CAD build for the part. Positions are in the model's coordinates, mm. Face numbers are marked on the shaded views. A direction names the side the tool comes from. Round coordinates to 2 decimals unless told otherwise and drop trailing zeros. Order: outer loops, then holes, each group sorted by start corner. A loop starts at its lowest first (then second) coordinate and runs counter-clockwise, first axis right, second up. Notation, with made-up numbers: M -23.5,84 L 12.5,84 A20 ccw 12.5,99 Z; hole C 4,4.5 d3. An arc over 180 degrees is marked long. Answer as a JSON object with one key per item and string values. Group by question number.
```python
from build123d import *

# Parameters (mm, degrees)
EXTRUDE_1_DEPTH     = 12.1
SKETCH_3_R          = 6.05
EXTRUDE_2_DEPTH     = 4.3
SKETCH_4_R          = 2.43
EXTRUDE_3_DEPTH     = 4
SKETCH_5_R          = 1.1
CUT_EXTRUDE_1_DEPTH = 4


with BuildPart() as part:
    # Эскиз1 → Бобышка-Вытянуть1 (new body)
    with BuildSketch(Plane.XY):
        Polygon((0, 0), (22.5, 0), (22.5, 15.7), (27.4, 15.7), (27.4, 18.2), (22.5, 18.2), (22.5, 22.4), (0, 22.4), (0, 18.2), (-4.9, 18.2), (-4.9, 15.7), (0, 15.7), align=None)
    extrude(amount=EXTRUDE_1_DEPTH)

    # Эскиз3 → Бобышка-Вытянуть2 (add)
    with BuildSketch(Plane(origin=(0, 22.4, 0), x_dir=(1, 0, 0), z_dir=(0, 1, 0))):
        with Locations(Location((16.45, -6.05, 0), (0, 0, 270))):
            Circle(SKETCH_3_R)
    extrude(amount=EXTRUDE_2_DEPTH)

    # Эскиз4 → Бобышка-Вытянуть3 (add)
    with BuildSketch(Plane(origin=(0, 26.7, 0), x_dir=(1, 0, 0), z_dir=(0, 1, 0))):
        with Locations(Location((16.45, -6.05, 0), (0, 0, 270))):
            Circle(SKETCH_4_R)
    extrude(amount=EXTRUDE_3_DEPTH)

    # Эскиз5 → Вырез-Вытянуть1 (cut)
    with BuildSketch(Plane(origin=(0, 18.2, 0), x_dir=(1, 0, 0), z_dir=(0, 1, 0))):
        with Locations(Location((25.1, -6.05, 0), (0, 0, 270))):
            Circle(SKETCH_5_R)
        with Locations(Location((-2.6, -6.05, 0), (0, 0, 270))):
            Circle(SKETCH_5_R)
    extrude(amount=-CUT_EXTRUDE_1_DEPTH, mode=Mode.SUBTRACT)


solid = part.part
```
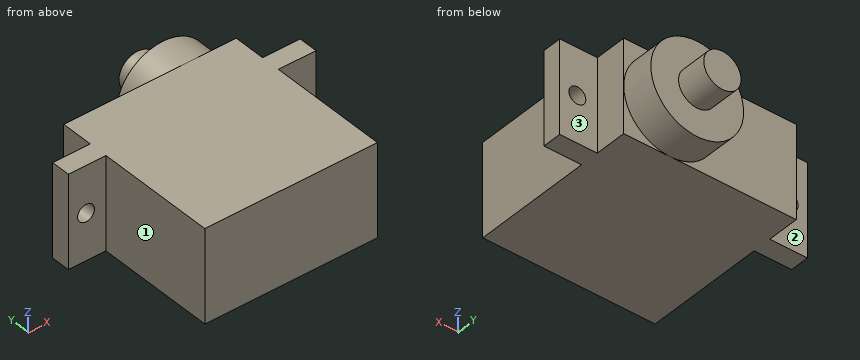
Item 1: Cut at B-B, the plane y = 16.5. Give the cut face in (x, z), and give its area (3 significant figures).
Item 2: Flat gauge pins, fed straight in: pin 1 Ø1.3 at (y, z) = (21.5, 4) entering from +X; pin 2 Ø5.5 at (x, z) = (-2, 5.5) entering from +Y; pin 3 Ø3 at (x, z) = (18.5, 9.5) entering from +Y. Where does each tip first touch, or does it go through?
Item 3: Drill centre lines: line 1 (X direction, y = 16.5, z = 6.05); line 2 (Z direction, x = 25, y = 17); line 3 (X direction, y = 6, z = 10). Where is each one in solid material? Low to high. Write a range as [from, to].
Item 4: Cut at A-A, the plane x = 25.1. Give the cut face in (y, z), and give its area (4 significant figures).
Item 5: Cut at C-C, the plane z = 1. Give the cut face in (x, y), and give its area (3 significant figures).
Item 6: Cut at D-D, the plane z = 6.75. Give the cut face in (x, y), and give its area (3 significant figures).
Item 7: 3-axis set-ups, long thin cutter, end or side, ignore diameter. For the marked faces 1, 2 and 3: which of +Z, -Z, +X, -X, +Y, -Y reach the whole face in a straight line?
Response values:
{
 "1": {"outline": "M -4.9,0 L 27.4,0 L 27.4,12.1 L -4.9,12.1 Z; hole C -2.6,6.05 d2.2; hole C 25.1,6.05 d2.2", "area": "383 mm^2"},
 "2": {"pin 1": "x = 22.5", "pin 2": "y = 22.4", "pin 3": "y = 26.7"},
 "3": {"line 1": "[-4.9, -3.7], [-1.5, 24], [26.2, 27.4]", "line 2": "[0, 4.95], [7.15, 12.1]", "line 3": "[0, 22.5]"},
 "4": {"outline": "M 15.7,0 L 18.2,0 L 18.2,4.95 L 15.7,4.95 Z; M 15.7,7.15 L 18.2,7.15 L 18.2,12.1 L 15.7,12.1 Z", "area": "24.75 mm^2"},
 "5": {"outline": "M -4.9,15.7 L 0,15.7 L 0,0 L 22.5,0 L 22.5,15.7 L 27.4,15.7 L 27.4,18.2 L 22.5,18.2 L 22.5,22.4 L 19.78,22.4 L 19.78,26.7 L 13.12,26.7 L 13.12,22.4 L 0,22.4 L 0,18.2 L -4.9,18.2 Z", "area": "557 mm^2"},
 "6": {"outline": "M -4.9,15.7 L -3.45,15.7 L -3.45,18.2 L -4.9,18.2 Z; M -1.75,15.7 L 0,15.7 L 0,0 L 22.5,0 L 22.5,15.7 L 24.25,15.7 L 24.25,18.2 L 22.5,18.2 L 22.5,22.4 L 22.46,22.4 L 22.46,26.7 L 18.78,26.7 L 18.78,30.7 L 14.12,30.7 L 14.12,26.7 L 10.44,26.7 L 10.44,22.4 L 0,22.4 L 0,18.2 L -1.75,18.2 Z; M 25.95,15.7 L 27.4,15.7 L 27.4,18.2 L 25.95,18.2 Z", "area": "590 mm^2"},
 "7": {"face 1": "+Z, -Z, -X, -Y", "face 2": "+Z, -Z, -X, +Y", "face 3": "+Z, -Z, +X, +Y"}
}
